Design review of the part shown in the three views and the two pictorial views. Dimensions are in mm from the part's minimum x, y and z. A direction names the side the tool comes from. Round coordinates to 2 decimals unless told otherwise and drop trailing zeros. Order: outer loops, then holes, each group sorted by start corner. A loop starts at its lowest first (then second) coordinate and runs counter-clockwise, first axis right, second up.
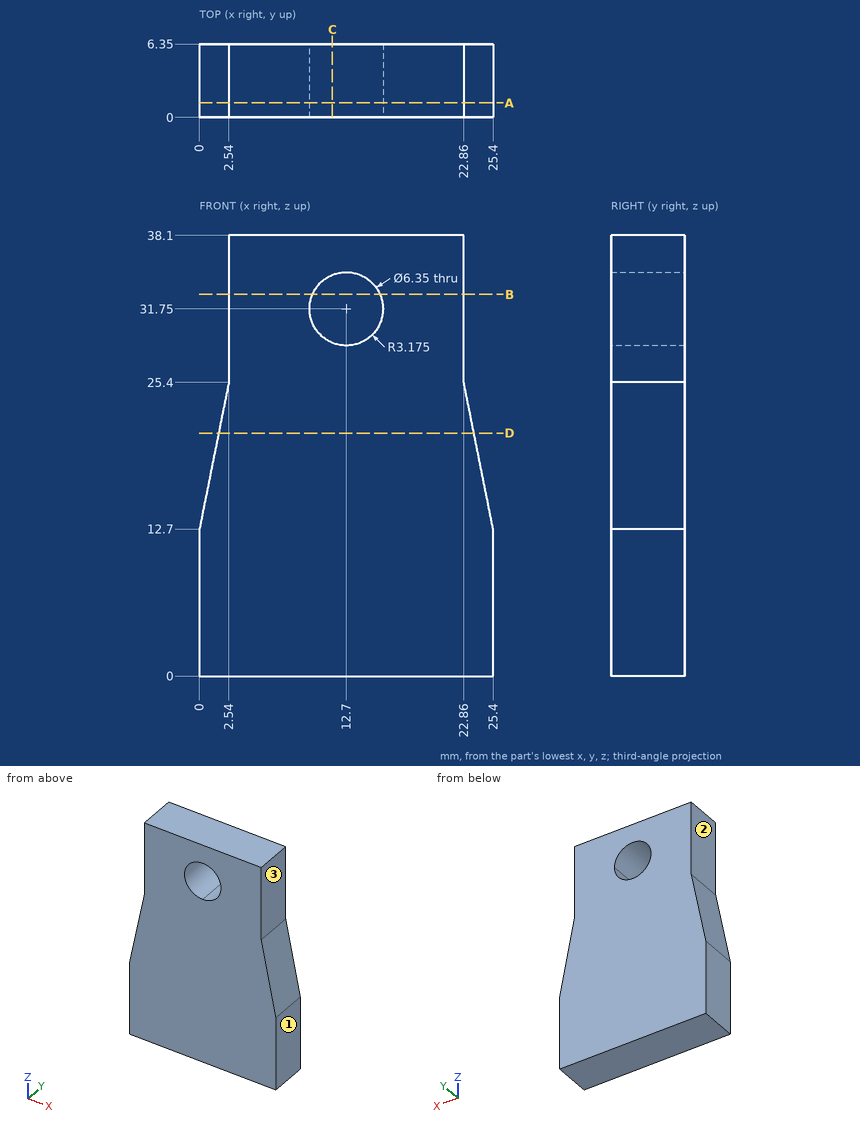
(1) Consider section D-D (z = 21). Write out the cut boundary in (x, y).
Data:
outline: (1.66, 0) - (23.74, 0) - (23.74, 6.35) - (1.66, 6.35) - close
(2) Consider section B-B (z = 33). Write out the cut boundary in (x, y).
Data:
outline: (2.54, 0) - (9.78, 0) - (9.78, 6.35) - (2.54, 6.35) - close; (15.62, 0) - (22.86, 0) - (22.86, 6.35) - (15.62, 6.35) - close
(3) Consider section C-C (x = 11.5). Write out the cut boundary in (y, z), and give its area (3 significant figures).
Data:
outline: (0, 0) - (6.35, 0) - (6.35, 28.81) - (0, 28.81) - close; (0, 34.69) - (6.35, 34.69) - (6.35, 38.1) - (0, 38.1) - close
area: 205 mm2
(4) Consider section A-A (y = 1.25). Write out the cut boundary in (x, z) (3 decimals), and give its area (3 significant figures).
Data:
outline: (0, 0) - (25.4, 0) - (25.4, 12.7) - (22.86, 25.4) - (22.86, 38.1) - (2.54, 38.1) - (2.54, 25.4) - (0, 12.7) - close; hole circle Ø6.35 at (12.7, 31.75)
area: 839 mm2
(5) To check wall thickness, follow probe 1 along X at (y, z) = (3.25, 31.75) (3 decimals); probe 2 along Z at (x, y) = (12.7, 2) (3 decimals); probe 3 along Z at (x, y) = (14.75, 5). State the ranges of each line that lie inside material, in increasing order.
Data:
probe 1: x = 2.54 to 9.525, 15.875 to 22.86
probe 2: z = 0 to 28.575, 34.925 to 38.1
probe 3: z = 0 to 29.33, 34.17 to 38.1
(6) For the marked faces 1, 2 and 3, list the 3-axis set-ups (+Z, -Z, +X, -X, +Y, -Y) from which the entire face can be reached by the end or side of a thin tool; tool diameter is ignored.
Data:
face 1: +Z, -Z, +X, +Y, -Y
face 2: +Z, -X, +Y, -Y
face 3: +Z, +X, +Y, -Y
(7) Insertion check: pin 1 (1.9 mm diameter, centred on y = 4, z = 29, fed in from -X); pin 2 (1 mm diameter, centred on y = 5.5, z = 21.5, fed in from -X); pin 3 (2 mm diameter, centred on y = 2.5, z = 19.5, fed in from +X). Each pin has a flat end and moves straight along its axis. Give the tip position at first contact, or say it passes through.
Data:
pin 1: stops at x = 2.54
pin 2: stops at x = 1.66
pin 3: stops at x = 24.24
